Can you work these out from the model? Positions are in its coordinate system, mm. A direction names the side the tool comes from. Give positions to 0.01 mm unless a question says otherwise; leave off trailing zeros. Write each loop counter-clockwise with the first axis right and the second up, starting at its lowest first coordinate (ties: lowest second). Pieces come first, ordered by that corner, then holes.
```python
from build123d import *

# Parameters (mm, degrees)
F0_W     = 238.125
F0_H     = 168.275
F1_DEPTH = 6.35
F2_R     = 5.08
F3_W     = 88.9
F3_H     = 88.9
F4_DEPTH = 25.4
F6_DEPTH = 25.4


with BuildPart() as f1:
    # F0 (on Top) → F1 (new body)
    with BuildSketch(Plane.XY):
        Rectangle(F0_W, F0_H)
    extrude(amount=F1_DEPTH)

    # F2
    f2_edges = [f1.edges().sort_by_distance(p)[0] for p in [
        (119.0625, 84.1375, 3.175),
        (-119.0625, 84.1375, 3.175),
        (119.0625, -84.1375, 3.175),
        (-119.0625, -84.1375, 3.175),
    ]]
    fillet(f2_edges, radius=F2_R)

    # F3 (on face) → F4 (cut)
    with BuildSketch(Plane.XY.offset(6.35)):
        Rectangle(F3_W, F3_H)
    extrude(amount=-F4_DEPTH, mode=Mode.SUBTRACT)

    # F5 (on face) → F6 (cut)
    with BuildSketch(Plane.XY.offset(6.35)):
        with BuildLine():
            ThreePointArc((45.72, 44.9326), (45.489376, 45.489376), (44.9326, 45.72))
            Line((44.9326, 45.72), (-44.9326, 45.72))
            ThreePointArc((-44.9326, 45.72), (-45.489376, 45.489376), (-45.72, 44.9326))
            Line((-45.72, 44.9326), (-45.72, -44.9326))
            ThreePointArc((-45.72, -44.9326), (-45.489376, -45.489376), (-44.9326, -45.72))
            Line((-44.9326, -45.72), (44.9326, -45.72))
            ThreePointArc((44.9326, -45.72), (45.489376, -45.489376), (45.72, -44.9326))
            Line((45.72, -44.9326), (45.72, 44.9326))
        make_face()
    extrude(amount=-F6_DEPTH, mode=Mode.SUBTRACT)


solid = f1.part
```
1) If we mould it in two halves opening along Y, with no side actions, what happens to faces 1 (the face through (-117.614, 82.61, 3.219)), 2 (the face through (-119.062, -1, 3)), 3 (the face through (-2, -84.138, 3)), 4 (the face through (1, 45.72, 3))? For each: +Y half, -Y half, draft (parallel to the pull), parting line (faces both ways), or undercut.
Values follow:
face 1: +Y half
face 2: draft
face 3: -Y half
face 4: undercut
2) Please list where these lines run through material, in increasing order: L1, parallel to Y at x = -3, z = 2.75; L2, parallel to X at y = 30, z = 3.
Values follow:
L1: y = -84.14 to -45.72, 45.72 to 84.14
L2: x = -119.06 to -45.72, 45.72 to 119.06
3) For faces 5 (the face through (45.72, -1, 3)), 6 (the face through (119.062, -1, 3)), which set-ups out of +Z, -Z, +X, -X, +Y, -Y let a thin tool reach every point of the face, with its end or its side?
Values follow:
face 5: +Z, -Z
face 6: +Z, -Z, +X, +Y, -Y
4) Suppose I cut it at B-B on y = 39.5. Write out the boundary of the cut face in (x, z), plus the area to 3 significant figures.
Values follow:
outline: (-119.06, 0) - (-45.72, 0) - (-45.72, 6.35) - (-119.06, 6.35) - close; (45.72, 0) - (119.06, 0) - (119.06, 6.35) - (45.72, 6.35) - close
area: 931 mm2
5) Suppose I cut it at C-C on z = 1. Write out the boundary of the cut face in (x, y).
Values follow:
outline: (-119.06, -79.06) arc R5.08 ccw to (-113.98, -84.14) - (113.98, -84.14) arc R5.08 ccw to (119.06, -79.06) - (119.06, 79.06) arc R5.08 ccw to (113.98, 84.14) - (-113.98, 84.14) arc R5.08 ccw to (-119.06, 79.06) - close; hole (-45.72, -44.93) arc R0.79 ccw to (-44.93, -45.72) - (44.93, -45.72) arc R0.79 ccw to (45.72, -44.93) - (45.72, 44.93) arc R0.79 ccw to (44.93, 45.72) - (-44.93, 45.72) arc R0.79 ccw to (-45.72, 44.93) - close
6) Suppose I cut it at A-A on x = -17.5. Write out the boundary of the cut face in (y, z).
Values follow:
outline: (-84.14, 0) - (-45.72, 0) - (-45.72, 6.35) - (-84.14, 6.35) - close; (45.72, 0) - (84.14, 0) - (84.14, 6.35) - (45.72, 6.35) - close
